Check sheet for the modelled part. Datum: model origin and axes. Units: mm. Face numbers are marked on the shaded views. A direction names the side the tool comes from. Coordinates: 2 decimals unless noted, no trailing zeros. Order: outer loops, then holes, each group sorted by start corner. A loop starts at its lowest first (then second) coordinate and runs counter-clockwise, first axis right, second up.
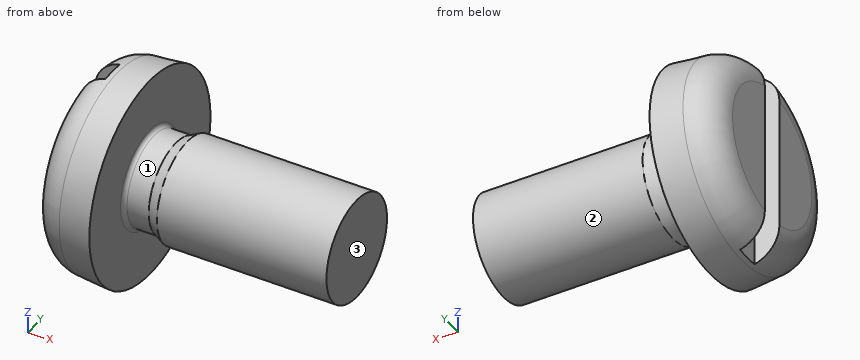
Autodesk Inventor part; units mm, degrees
ref_plane "Work Plane1" through (30.1625, 0, 0) normal (0, 0, -1) x (1, 0, 0)
ref_plane "YZ Plane" through (0, 0, 0) normal (1, 0, 0) x (0, 1, 0)
ref_plane "XZ Plane" through (0, 0, 0) normal (0, 1, 0) x (-1, 0, 0)
sketch "Skizze1" plane through (0, 0, 0) normal (0, 0, 1) x (1, 0, 0)
  line L0 (-1.5, 0) -> (5, 0)
  line L1 (5, 0) -> (5, 1.25)
  line L2 (5, 1.25) -> (0.9, 1.25)
  line L3 (0.9, 1.25) -> (0.6238, 1.112)
  line L4 (0.6238, 1.112) -> (0, 1.112)
  line L5 (0, 1.112) -> (0, 2.5)
  line L6 (-2.8, 0) -> (6.3, 0)
  line L7 (0, -0.5) -> (0, 3)
  line L8 (-1.5, 0) -> (-1.5, 2.3688)
  line L9 (0, 2.5) -> (-1.5, 2.3688)
  line L10 (0.9, 1.25) -> (0, 1.25) construction
  dimension "d0" = 5
  dimension "d1" = 4.1
  dimension "d2" = 0.2762
  dimension "d3" = 1.5
  dimension "d4" = 2.5
  dimension "d5" = 2.224
  dimension "d9" = 5
  dimension "d10" = 5
revolve "Körper" add sketch "Skizze1" angle 360 about axis through (-1.5, 0, 0) along (1, 0, 0)
sketch "Skizze2" plane through (-1.5, 0, 0) normal (-1, 0, 0) x (0, 0, 1)
  circle A0 centre (0, 0) radius 2.5
  line L0 (0, 0) -> (0, 2.3688)
  line L1 (-2.5, 0.3) -> (2.5, 0.3)
  line L2 (2.5, 0.3) -> (2.5, -0.3)
  line L3 (2.5, -0.3) -> (-2.5, -0.3)
  line L4 (-2.5, -0.3) -> (-2.5, 0.3)
  line L5 (-2.5, 0) -> (2.5, 0) construction
  line L6 (0, 0.3) -> (0, -0.3) construction
  dimension "d11" = 0.6
  dimension "d12" = 5
fillet "Rundung1" radius 0.8 1 edges at (-1.5, -2.3688, 0)
extrude "Loch" cut sketch "Skizze2" against normal blind 0.6 contours A0 L3 L1 | L2 L3 A0 | A0 L1 L2 | A0 L4 L1 | L3 L4 A0
thread "Gewinde"
ref_plane "Work Plane1" through (30.1625, 0, 0) normal (0, 0, -1) x (1, 0, 0)
fillet "Fillet5" radius 0.1 1 edges at (0, -1.112, 0)
equation "\"d11\" = SBR"
equation "\"d12\" = KOD"
equation "\"d14\" = RR"
equation "\"d19\" = STI"
equation "\"d15\" = GEL"
equation "\"d41\" = R"
equation "\"d0\" = NLG"
equation "\"d1\" = GEL"
equation "\"d3\" = KOH"
equation "\"d4\" = GD"
equation "\"d5\" = BDM"
equation "\"d9\" = KOD"
equation "\"d10\" = KEWI"
equation "\"GD\" = NND"
equation "\"NLG\" = 5"
equation "\"GEL\" = 4.1"
equation "\"KOD\" = 5"
equation "\"KOH\" = 1.5"
equation "\"GAL\" = 0.61345 * PTC"
equation "\"R\" = 0.1"
equation "\"BDM\" = 2.224"
equation "\"GUL\" = 0.61345 * PTC"
equation "\"RR\" = 0.8"
equation "\"SBR\" = 0.6"
equation "\"STI\" = 0.6"
equation "\"KEWI\" = 5deg"
equation "\"PTC\" = 0.45"
equation "\"THREADDIA\" = 2.5"
equation "\"TOA\" = 30deg"
equation "\"NND\" = 2.5"
equation "\"GD1\" = THREADDIA - 1.2269 * PTC"
properties part number "ISO 1580 - M2,5 x 5" material "Stahl, weich"
(1) Cross-section at B-B (z = 0). Enter the section's corners in (x, y).
Filled in:
outline: (-1.5, -1.64) arc R0.8 ccw to (-0.77, -2.43) - (0, -2.5) - (0, -1.21) arc R0.1 cw to (0.1, -1.11) - (0.62, -1.11) - (0.9, -1.25) - (5, -1.25) - (5, 1.25) - (0.9, 1.25) - (0.62, 1.11) - (0.1, 1.11) arc R0.1 cw to (0, 1.21) - (0, 2.5) - (-0.77, 2.43) arc R0.8 ccw to (-1.5, 1.64) - (-1.5, 0.3) - (-0.9, 0.3) - (-0.9, -0.3) - (-1.5, -0.3) - close
(2) Cross-section at A-A (y = 0). Enter the section's corners in (x, z), and give its area (3 significant figures).
Filled in:
outline: (-0.9, -2.41) arc R0.8 ccw to (-0.77, -2.43) - (0, -2.5) - (0, -1.21) arc R0.1 cw to (0.1, -1.11) - (0.62, -1.11) - (0.9, -1.25) - (5, -1.25) - (5, 1.25) - (0.9, 1.25) - (0.62, 1.11) - (0.1, 1.11) arc R0.1 cw to (0, 1.21) - (0, 2.5) - (-0.77, 2.43) arc R0.8 ccw to (-0.9, 2.41) - close
area: 16.7 mm2
(3) Cross-section at C-C (x = 4). Enter the section's corners in (y, z).
Filled in:
outline: circle Ø2.5 at (0, 0)
(4) Go/stop test with flat-tipped pins: P1, Ø1.5, axis at x = 3, y = 1.5, coming from the -Z side; P2, Ø0.5, axis at x = -1, z = -1, coming from the -Y side; P3, Ø0.5, axis at y = 0, z = 0, coming from the -X side; P4, Ø2, axis at y = 1.5, z = -1.5, coming from the +X side. Record where each tip stops, or that it passes through.
Filled in:
P1: stops at z = -1
P2: stops at y = -2.29
P3: stops at x = -0.9
P4: stops at x = 5
(5) Thickness scan on probe 1 along X at (y, z) = (-0.25, -0.4); probe 2 along X at (y, z) = (-1.6, 0.05); probe 3 along Y at (x, z) = (2.5, 0.4). Record the ranges inside material, lowest first.
Filled in:
probe 1: x = -0.9 to 5
probe 2: x = -1.5 to 0
probe 3: y = -1.18 to 1.18
(6) Tool access check on the marked faces 1, 2 and 3. Record the directions out of +Z, -Z, +X, -X, +Y, -Y that give a thin tool (end or side, any length) a straight path to the whole face; none if there is none.
Filled in:
face 1: none
face 2: +X
face 3: +Z, -Z, +X, +Y, -Y
